Read the model definition and answer for the solid it produces. Units are mm, in the model's axes. Coordinates: 2 decimals unless noted, no trailing zeros. Loops run counter-clockwise (first coordinate to the right, second up) from the corner with the lowest first, then second, coordinate; pieces in that order, holes last. Notation, with made-up numbers: M -35,72 L -12,72 A20 ccw -12,97 Z; hole C 19.25,-7.75 d9. An arc over 180 degrees is marked long. Use one line per item in the form item = value. Start each with the question number.
1. The part is cut by section A-A (y = 3.05). Give the vertices of the cut face in (x, z).
2. The part is cut by section B-B (z = -7.5). Give the vertices of the cut face in (x, y), plus the area to 3 significant figures.
3. Flat-ended cylindrical pins translate along their axes: pin 1 (5 mm diameter, centred on x = 16, z = -4, fed in from -Y); pin 2 (2 mm diameter, centred on x = -37.5, y = 3, fed in from -Z). Find the tip coordinate at first contact, or state that the pin passes through.
4. Find the intervals of material crossed by probe 1 along X at (y, z) = (0.6, -3); probe 2 along Z at (x, y) = (-39, 1.45), in increasing order. Write a range as [from, to].
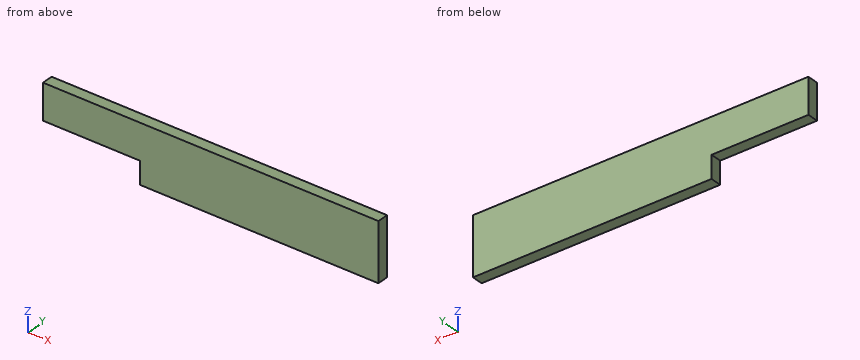
from build123d import *

# Parameters (mm, degrees)
SKETCH1_W               = 121
SKETCH1_H               = 21
BOSS_EXTRUDE1_DEPTH     = 4
CUT_EXTRUDE1_DEPTH      = 62.534543144
CUT_EXTRUDE1_DEPTH_BACK = 62.534543144
SKETCH2_W               = 36.59359186
SKETCH2_H               = 8.142757597


with BuildPart() as part:
    # Sketch1 → Boss-Extrude1 (new body)
    with BuildSketch(Plane(origin=(0, 0, 0), x_dir=(1, 0, 0), z_dir=(0, 1, 0))):
        Rectangle(SKETCH1_W, SKETCH1_H)
    extrude(amount=BOSS_EXTRUDE1_DEPTH)

    # Sketch2 → Cut-Extrude1 (cut, two sides: drawn at the far end of the back side and taken through both)
    with BuildSketch(Plane(origin=(0, 0, 0), x_dir=(1, 0, 0), z_dir=(0, 1, 0)).offset(-CUT_EXTRUDE1_DEPTH_BACK)):
        with Locations((-43.854273263, 6.428621202)):
            Rectangle(SKETCH2_W, SKETCH2_H)
    extrude(amount=CUT_EXTRUDE1_DEPTH + CUT_EXTRUDE1_DEPTH_BACK, mode=Mode.SUBTRACT)


solid = part.part
Computed values:
q1.outline = M -60.5,-2.36 L -25.56,-2.36 L -25.56,-10.5 L 60.5,-10.5 L 60.5,10.5 L -60.5,10.5 Z
q2.outline = M -25.56,0 L 60.5,0 L 60.5,4 L -25.56,4 Z
q2.area = 344 mm²
q3.pin_1 = 0
q3.pin_2 = -2.36
q4.probe_1 = [-25.56, 60.5]
q4.probe_2 = [-2.36, 10.5]
